Could you check a few things on this model? Use its own coordinates, in mm. Face numbers are marked on the shaded views. A direction names the side the tool comes from. Give positions to 0.01 mm unless a question says otherwise; leave off trailing zeros. Loops run counter-clockwise (first coordinate to the right, second up) from the corner with the lowest first, then second, coordinate; pieces in that order, holes last. Notation, with made-up numbers: M 11,-10 L 47,-10 A37 ccw 47,29 Z; hole C 74.5,48 d9. An arc over 180 degrees is marked long. Return JSON: item names as keys, results as strings. Group by question number.
1. Please list where these lines run through material, in increasing order: line 1 (X direction, y = 3.5, z = 2.7); line 2 (Y direction, x = 0, z = 1.3); line 3 (X direction, y = 2.5, z = 0.85).
2. For pin 1 (3 mm diameter, centred on x = 40, y = 0, fed in from +Z); pin 2 (0.8 mm diameter, centred on y = -4.5, z = 4.5, fed in from -X); pin 3 (12 mm diameter, centred on x = -2.5, y = -7, fed in from +Z), each with a flat end and sliding along its axis, tell me the tip position at first contact or that it passes through.
3. If we mould it in two halves opening along Y, with no side actions, what happens to the marked faces 3, 4 and 5? For each: +Y half, -Y half, draft (parallel to the pull), parting line (faces both ways), or undercut.
4. If we section it at A-A (x = 0): Write out the boundary of the cut face in (y, z), plus the area to 3 significant figures.
5. If we section it at C-C (x = 17): Write out the boundary of the cut face in (y, z), plus the area to 3 significant figures.
6. For the marked faces 1 and 2, which set-ups out of +Z, -Z, +X, -X, +Y, -Y let a thin tool reach every point of the face, with its end or its side?
7. If we section it at B-B (y = 0): State how many separate pieces and enclosed holes the cut face has, plus the area to 3 significant figures.
```python
from build123d import *

# Parameters (mm, degrees)
SKETCH_1_W          = 90
SKETCH_1_H          = 20
EXTRUDE_1_DEPTH     = 4
SKETCH_2_W          = 13
SKETCH_2_H          = 20
EXTRUDE_2_DEPTH     = 1
SKETCH_4_R          = 5.1
EXTRUDE_3_DEPTH     = 4
SKETCH_3_R          = 1.8
CUT_EXTRUDE_1_DEPTH = 47.270941205
SKETCH_4_3_R        = 5.1
CUT_EXTRUDE_3_DEPTH = 47.270941205
SKETCH_7_OUTSIDE_W  = 110.466
SKETCH_7_OUTSIDE_H  = 40.466
CUT_EXTRUDE_6_DEPTH = 10
CUT_EXTRUDE_7_DEPTH = 47.368092477
CUT_EXTRUDE_8_DEPTH = 47.270941205
FILLET_1_R          = 1


with BuildPart() as part:
    # ｽｹｯﾁ1 → ﾎﾞｽ - 押し出し1 (new body)
    with BuildSketch(Plane.XY):
        Rectangle(SKETCH_1_W, SKETCH_1_H)
    extrude(amount=EXTRUDE_1_DEPTH)

    # ｽｹｯﾁ2 → ﾎﾞｽ - 押し出し2 (add)
    with BuildSketch(Plane.XY.offset(4)):
        with Locations((-28.5, 0)):
            Rectangle(SKETCH_2_W, SKETCH_2_H)
        with Locations((28.5, 0)):
            Rectangle(SKETCH_2_W, SKETCH_2_H)
    extrude(amount=EXTRUDE_2_DEPTH)

    # ｽｹｯﾁ4 → ﾎﾞｽ - 押し出し3 (add)
    with BuildSketch(Plane.XY.offset(4)):
        Circle(SKETCH_4_R)
    extrude(amount=-EXTRUDE_3_DEPTH)

    # ｽｹｯﾁ3 → ｶｯﾄ - 押し出し1 (cut, through all)
    with BuildSketch(Plane.XY.offset(4)):
        with Locations((-40, 0)):
            Circle(SKETCH_3_R)
        with Locations((-17, 0)):
            Circle(SKETCH_3_R)
        with Locations((17, 0)):
            Circle(SKETCH_3_R)
        with Locations((40, 0)):
            Circle(SKETCH_3_R)
    extrude(amount=-CUT_EXTRUDE_1_DEPTH, mode=Mode.SUBTRACT)

    # ｽｹｯﾁ4<3> → ｶｯﾄ - 押し出し3 (cut, through all)
    with BuildSketch(Plane.XY.offset(4)):
        Circle(SKETCH_4_3_R)
    extrude(amount=-CUT_EXTRUDE_3_DEPTH, mode=Mode.SUBTRACT)

    # ｽｹｯﾁ7 outside → ｶｯﾄ - 押し出し6 (cut)
    with BuildSketch(Plane(origin=(0, 0, 0), x_dir=(-1, 0, 0), z_dir=(0, 0, -1))):
        Rectangle(SKETCH_7_OUTSIDE_W, SKETCH_7_OUTSIDE_H)
        Polygon((-45, 5), (-45, -5), (-12, -10), (12, -10), (45, -5), (45, 5), (12, 10), (-12, 10), align=None, mode=Mode.SUBTRACT)
    extrude(amount=-CUT_EXTRUDE_6_DEPTH, mode=Mode.SUBTRACT)

    # ｽｹｯﾁ8 → ｶｯﾄ - 押し出し7 (cut, through all)
    with BuildSketch(Plane.XY.offset(5)):
        Polygon((22, 5.450608618), (22, -5.450608618), (35, -3.480911648), (35, 3.480911648), align=None)
        Polygon((-22, 5.450608618), (-35, 3.480911648), (-35, -3.480911648), (-22, -5.450608618), align=None)
    extrude(amount=-CUT_EXTRUDE_7_DEPTH, mode=Mode.SUBTRACT)

    # ｽｹｯﾁ9 → ｶｯﾄ - 押し出し8 (cut, through all)
    with BuildSketch(Plane.XY.offset(4)):
        with BuildLine():
            Line((-12, 6.837276926), (-12, -7))
            Line((-12, -7), (-3.872983346, -7))
            ThreePointArc((-3.872983346, -7), (-7.998356489, -0.162152651), (-4.153509869, 6.837276926))
            Line((-4.153509869, 6.837276926), (-12, 6.837276926))
        make_face()
        with BuildLine():
            Line((4.153509869, 6.837276926), (12, 6.837276926))
            Line((12, 6.837276926), (12, -7))
            Line((12, -7), (3.872983346, -7))
            ThreePointArc((3.872983346, -7), (7.998356489, -0.162152651), (4.153509869, 6.837276926))
        make_face()
    extrude(amount=-CUT_EXTRUDE_8_DEPTH, mode=Mode.SUBTRACT)

    # ﾌｨﾚｯﾄ1
    fillet_1_edges = [part.edges().sort_by_distance(p)[0] for p in [
        (22, 5.450608618, 2),
        (35, 3.480911648, 2),
        (35, -3.480911648, 2),
        (22, -5.450608618, 2),
        (-22, 5.450608618, 2),
        (-22, -5.450608618, 2),
        (-35, -3.480911648, 2),
        (-35, 3.480911648, 2),
        (-12, 6.837276926, 2),
        (-4.153509869, 6.837276926, 2),
        (-3.872983346, -7, 2),
        (-12, -7, 2),
        (12, -7, 2),
        (3.872983346, -7, 2),
        (4.153509869, 6.837276926, 2),
        (12, 6.837276926, 2),
    ]]
    fillet(fillet_1_edges, radius=FILLET_1_R)


solid = part.part
```
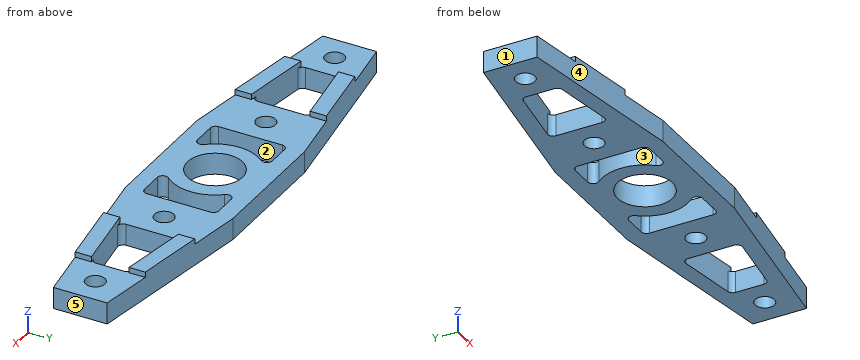
Answer:
{
 "1": {"line 1": "x = -45 to -34.48, -22 to -12, -7.19 to -3.71, 3.71 to 7.19, 12 to 22, 34.48 to 45", "line 2": "y = -10 to -5.1, 5.1 to 10", "line 3": "x = -45 to -35, -22 to -12, -7.6 to -4.45, 4.45 to 7.6, 12 to 22, 35 to 45"},
 "2": {"pin 1": "passes through", "pin 2": "stops at x = -35", "pin 3": "stops at z = 4"},
 "3": {"face 3": "undercut", "face 4": "-Y half", "face 5": "draft"},
 "4": {"outline": "M -10,0 L -5.1,0 L -5.1,4 L -10,4 Z; M 5.1,0 L 10,0 L 10,4 L 5.1,4 Z", "area": "39.2 mm²"},
 "5": {"outline": "M -9.24,0 L -1.8,0 L -1.8,4 L -9.24,4 Z; M 1.8,0 L 9.24,0 L 9.24,4 L 1.8,4 Z", "area": "59.5 mm²"},
 "6": {"face 1": "+Z, -Z, -X, +Y, -Y", "face 2": "+Z, -Z"},
 "7": {"separate pieces": "10", "enclosed holes": "0", "area": "126 mm²"}
}
